The drawing under review shows one solid part. Ordinate dimensions are in mm from its lowest x, y, z. A direction names the side the tool comes from. Coordinates: 2 decimals unless noted, no trailing zeros. Write each loop counter-clockwise with the first axis right and the second up, starting at its lowest first coordinate (ties: lowest second). Pieces come first, ordered by that corner, then holes.
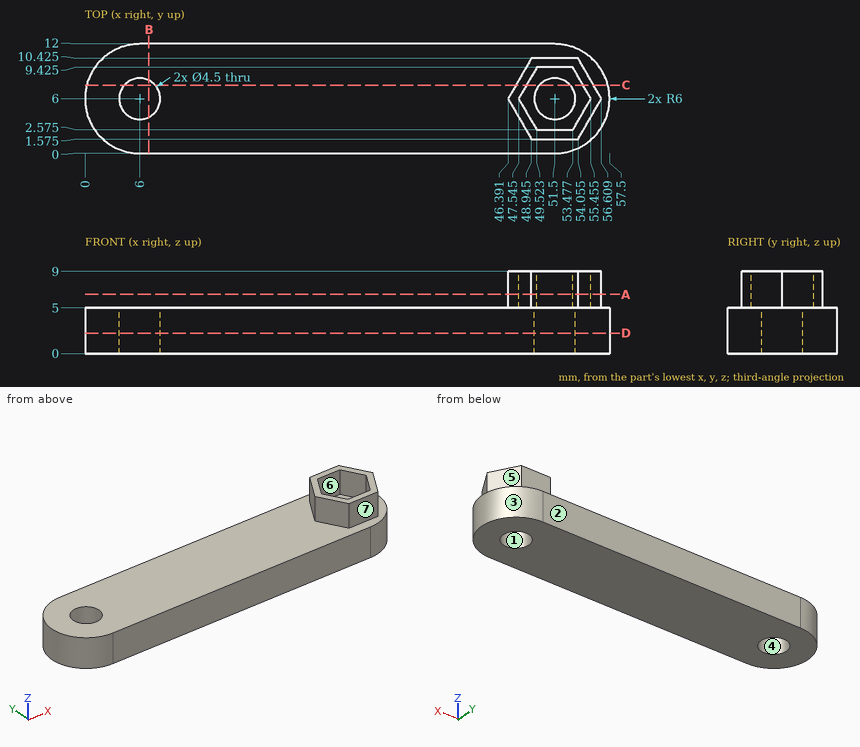
Q1. For probe 1 along X at (y, z) = (6, 1.9); probe 2 along Y at (x, z) = (6, 2.7); probe 3 along Z at (x, y) = (3.5, 10.25), list the stretches that pass through material, from the lowest coordinate up.
Ans:
probe 1: x = 0 to 3.75, 8.25 to 49.25, 53.75 to 57.5
probe 2: y = 0 to 3.75, 8.25 to 12
probe 3: z = 0 to 5
Q2. Clearance check with flat-ended pins moving along their axes: pin 1 Ø1.2 at (x, z) = (52, 7.5) entering from -Y (1 decimal); pin 2 Ø4.5 at (x, z) = (51.5, 7.5) entering from +Y (1 decimal); pin 3 Ø4 at (x, y) = (46, 1.5) entering from +Z. State where each tip first meets the part, or that it passes through.
Ans:
pin 1: stops at y = 1.6
pin 2: stops at y = 10.4
pin 3: stops at z = 5
Q3. Add section B-B (x = 7). State the section outline as (y, z) points (1 decimal).
Ans:
outline: (0, 0) - (4, 0) - (4, 5) - (0, 5) - close; (8, 0) - (12, 0) - (12, 5) - (8, 5) - close
Q4. Tool access review of the marked faces 5, 6 and 7: name each direction out of +Z, -Z, +X, -X, +Y, -Y from which nothing blocks a thin tool from reaching the whole face with its end or side.
Ans:
face 5: +Z, +X, +Y
face 6: +Z
face 7: +Z, +X, -X, -Y
Q5. Add section A-A (z = 6.5). State the section outline as (x, y) points (1 decimal).
Ans:
outline: (46.4, 6) - (48.9, 1.6) - (54.1, 1.6) - (56.6, 6) - (54.1, 10.4) - (48.9, 10.4) - close; hole (47.5, 6) - (49.5, 2.6) - (53.5, 2.6) - (55.5, 6) - (53.5, 9.4) - (49.5, 9.4) - close
Q6. Add section C-C (y = 7.5). State the section outline as (x, z) points.
Ans:
outline: (0.19, 0) - (4.32, 0) - (4.32, 5) - (0.19, 5) - close; (7.68, 0) - (49.82, 0) - (49.82, 5) - (48.41, 5) - (48.41, 9) - (47.26, 9) - (47.26, 5) - (7.68, 5) - close; (53.18, 0) - (57.31, 0) - (57.31, 5) - (55.74, 5) - (55.74, 9) - (54.59, 9) - (54.59, 5) - (53.18, 5) - close
Q7. Add section D-D (z = 2.25). State the section outline as (x, y) points, then the cut area to 3 significant figures.
Ans:
outline: (6, 0) - (51.5, 0) arc R6 ccw to (51.5, 12) - (6, 12) arc R6 ccw to start; hole circle Ø4.5 at (6, 6); hole circle Ø4.5 at (51.5, 6)
area: 627 mm2
Q8. Draft analysis for pull direction X (two halves, no side actions). For the marked faces 1, 2, 3 and 4, state which applies: +X half, -X half, draft (parallel to the pull), parting line (faces both ways), or undercut.
Ans:
face 1: undercut
face 2: draft
face 3: +X half
face 4: undercut
